The model under review builds one solid part; all positions refer to its coordinate system, in mm. A direction names the side the tool comes from. Coordinates: 2 decimals unless noted, no trailing zeros. One line per item, written item: value. Start each with the question number.
1. For faces 1 (the face through (-107.971, 55.173, 20.21)), 2 (the face through (-109.576, -23.177, 20.21)), 3 (the face through (-66.157, -101.612, 20.21)), list the 3-axis set-ups (+Z, -Z, +X, -X, +Y, -Y) from which the entire face can be reached by the end or side of a thin tool; tool diameter is ignored.
2. We need section A-A, the plane x = -15. Count the separate pieces of the cut face and the enclosed holes in it, then the cut area to 3 significant figures.
3. Mouldability with a two-part tool opening along Y and no side actions: class faces 4 (the face through (-66.067, 101.374, 20.21)), 5 (the face through (-55.85, 36.5, 20.07)), 6 (the face through (93.91, 76.3, 20.21)), 7 (the face through (-96.689, -86.898, 20.21)) as +Y half, -Y half, draft (parallel to the pull), parting line (faces both ways), or undercut.
4. Insertion check: P1, Ø1.5, axis at y = -98.5, z = 5.5, coming from the +X side; P2, Ø10, axis at x = -65, z = 11.5, coming from the -Y side; P3, Ø10, axis at y = 34.5, z = 27.5, coming from the -X side; P4, Ø6, axis at x = -60.62, y = 35, coming from the -Z side. Each pin has a flat end and moves straight along its axis. Give the tip position at first contact, or say it passes through.
5. To check wall thickness, follow line 1 (Y direction, x = 0, z = 31); line 2 (X direction, y = 71.5, z = 12); line 3 (Y direction, x = 21, z = 27). State the ranges of each line that lie inside material, in increasing order.
from build123d import *

# Parameters (mm, degrees)
FILLET_1_R               = 5
CHAMFER_1_SIZE           = 1
CUT_EXTRUDE_2_DEPTH      = 189.148877222
PATTERN_CIRCULAR_1_COUNT = 30
SKETCH_4_R               = 5
CUT_EXTRUDE_3_DEPTH      = 189.081998408


with BuildPart() as part:
    # Sketch 1 → Revolve 1 (revolve)
    with BuildSketch(Plane(origin=(0, 0, 0), x_dir=(1, 0, 0), z_dir=(0, 1, 0)), mode=Mode.PRIVATE) as revolve_1_sk:
        Polygon((20, 0), (45, 0), (45, -15), (100, -15), (100, -5), (130, -5), (130, -35), (100, -35), (100, -25), (45, -25), (45, -40), (20, -40), align=None)
    revolve(revolve_1_sk.sketch.rotate(Axis((0, 0, 0), (0, 0, 1)), 180), axis=Axis((0, 0, 0), (0, 0, 1)))

    # Fillet 1
    fillet_1_edges = [part.edges().sort_by_distance(p)[0] for p in [
        (45, 0, 25),
        (100, 0, 25),
        (100, 0, 15),
        (45, 0, 15),
    ]]
    fillet(fillet_1_edges, radius=FILLET_1_R)

    # Chamfer 1
    chamfer_1_edges = [part.edges().sort_by_distance(p)[0] for p in [
        (20, 0, 0),
        (20, 0, 40),
    ]]
    chamfer(chamfer_1_edges, length=CHAMFER_1_SIZE)

    # Sketch 3 → Cut-Extrude 2 (cut, through all)
    with BuildSketch(Plane.XY.offset(40)):
        Polygon((112, 8), (135, 4.1667), (135, -4.1667), (112, -8), align=None)
    cut_extrude_2 = extrude(amount=-CUT_EXTRUDE_2_DEPTH, mode=Mode.SUBTRACT)

    # Pattern Circular 1: Cut-Extrude 2 ×30 about axis
    pattern_circular_1_axis = Axis((0, 0, 0), (0, 0, 1))
    for i in range(1, PATTERN_CIRCULAR_1_COUNT):
        add(cut_extrude_2.rotate(pattern_circular_1_axis, i * 360 / PATTERN_CIRCULAR_1_COUNT), mode=Mode.SUBTRACT)

    # Sketch 4 → Cut-Extrude 3 (cut, through all)
    with BuildSketch(Plane.XY.offset(40)):
        with Locations((69.616533, 7.316992)):
            Circle(SKETCH_4_R)
        with Locations((52.020138, 46.839142)):
            Circle(SKETCH_4_R)
        with Locations((14.553818, 68.470332)):
            Circle(SKETCH_4_R)
        with Locations((-28.471565, 63.948182)):
            Circle(SKETCH_4_R)
        with Locations((-60.621778, 35)):
            Circle(SKETCH_4_R)
        with Locations((-69.616533, -7.316992)):
            Circle(SKETCH_4_R)
        with Locations((-52.020138, -46.839142)):
            Circle(SKETCH_4_R)
        with Locations((-14.553818, -68.470332)):
            Circle(SKETCH_4_R)
        with Locations((28.471565, -63.948182)):
            Circle(SKETCH_4_R)
        with Locations((60.621778, -35)):
            Circle(SKETCH_4_R)
    extrude(amount=-CUT_EXTRUDE_3_DEPTH, mode=Mode.SUBTRACT)


solid = part.part
Findings below:
1. face 1: +Z, -Z, -X
1. face 2: +Z, -Z
1. face 3: +Z, -Z, -Y
2. separate pieces: 3
2. enclosed holes: 0
2. area: 4,140 mm2
3. face 4: +Y half
3. face 5: undercut
3. face 6: undercut
3. face 7: -Y half
4. P1: x = 82.39
4. P2: y = -115.33
4. P3: x = -126.02
4. P4: through
5. line 1: -130 to -100, -45 to -20, 20 to 45, 100 to 130
5. line 2: -108.57 to -107.26, -86.49 to -69.31, 69.31 to 86.49, 107.26 to 108.57
5. line 3: -128.29 to -96.75, -40.93 to 40.93, 96.75 to 128.29
